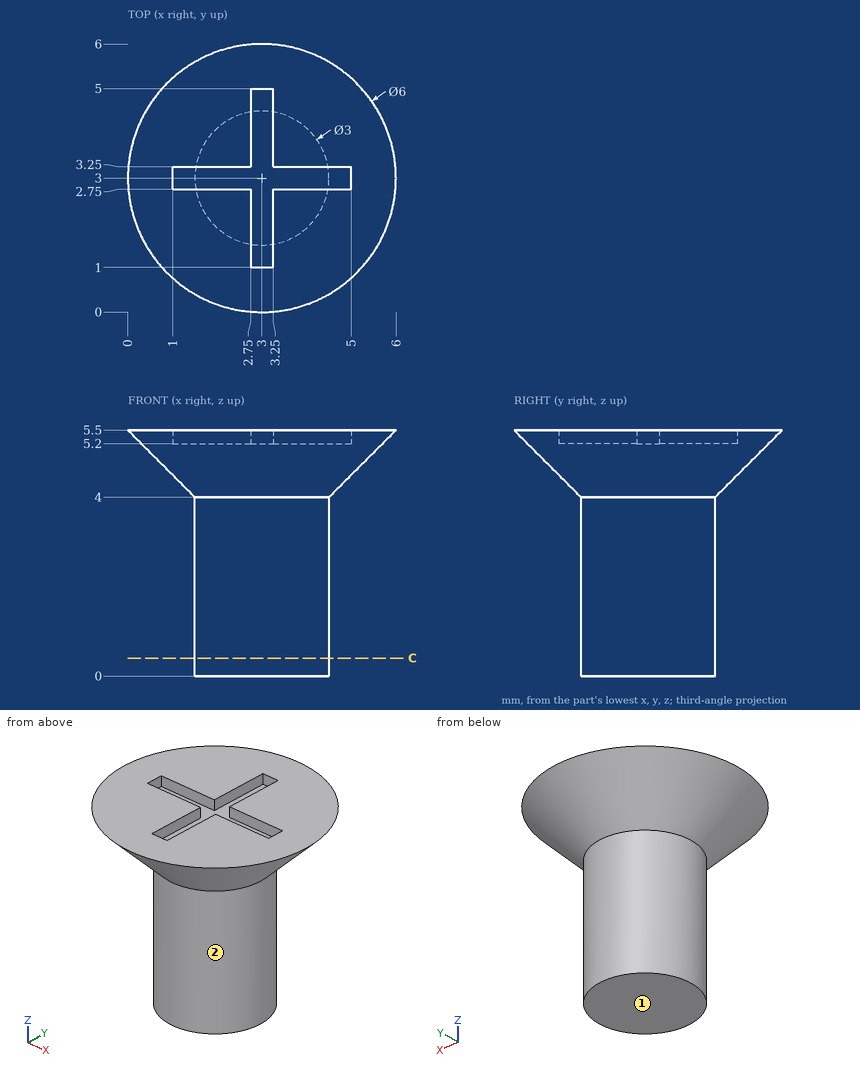
Input: dimensioned drawing with shaded views. Units: mm. Origin: part minimum x, y, z. Give positions to 0.01 mm unless a question says otherwise; leave off trailing zeros. Write each loop counter-clockwise with the first axis right and the second up, starting at its lowest first coordinate (ties: lowest second). Pieces come first, ordered by that corner, then holes.
1. First-contact query: pin 1 (3 mm diameter, centred on x = 2, z = 2, fed in from -Y); pin 2 (1.5 mm diameter, centred on x = 3.5, z = 0.5, fed in from +Y); pin 3 (2 mm diameter, centred on y = 1.5, z = 0.5, fed in from +X). Flat tips, straight axial feed; report the tip coordinate or a pass-through.
2. Material intervals for line 1 along Z through (x, y) = (3.15, 3.6); line 2 along X through (y, z) = (1.85, 0.4); line 3 along Y through (x, z) = (4.7, 4.6), sorted ascending.
3. Section query C-C (z = 0.4). Return the cut outline in (x, y), then the cut area to 3 significant figures.
4. Pull-direction query (Y, two-part tool) for the marked faces 1 and 2; classes: +Y half, -Y half, draft (parallel to the pull), parting line (faces both ways), or undercut.
Output values:
1. pin 1: stops at y = 1.5
1. pin 2: stops at y = 4.5
1. pin 3: stops at x = 4.41
2. line 1: z = 0 to 5.2
2. line 2: x = 2.04 to 3.96
2. line 3: y = 1.77 to 4.23
3. outline: circle Ø3 at (3, 3)
3. area: 7.07 mm2
4. face 1: draft
4. face 2: parting line
